from build123d import *

# Parameters (mm, degrees)
BOSS_EXTRUDE1_DEPTH = 1.6


with BuildPart() as part:
    # Эскиз1 → Повернуть1 (revolve)
    with BuildSketch(Plane.XY):
        Polygon((-2.875, 1.8), (0, 1.8), (0, -11.24), (-0.65, -11.9), (-1.195, -11.9), (-1.5, -11.595), (-1.5, -4.645), (-1.195, -4.34), (-1.195, 1), (-2.5, 1), (-2.5, 0), (-2.925, 0), (-2.925, 1.75), align=None)
    revolve(axis=Axis((0, 0, 0), (0, -1, 0)))

    # Sketch1 → Boss-Extrude1 (add)
    with BuildSketch(Plane(origin=(0, 1.8, 0), x_dir=(1, 0, 0), z_dir=(0, 1, 0))):
        Polygon((1.688749537, 2.925), (-1.688749537, 2.925), (-3.377499075, 0), (-1.688749537, -2.925), (1.688749537, -2.925), (3.377499075, 0), align=None)
    extrude(amount=-BOSS_EXTRUDE1_DEPTH)


solid = part.part
Verification items for the finished model (mm, model axes). A direction names the side the tool comes from. Coordinates: 2 decimals unless noted, no trailing zeros. Order: outer loops, then holes, each group sorted by start corner. A loop starts at its lowest first (then second) coordinate and runs counter-clockwise, first axis right, second up. Notation, with made-up numbers: (-26, -14.5) -> (21, -14.5) arc R19 ccw to (21, 4.5) -> close; hole circle Ø7 at (11, -26). An arc over 180 degrees is marked (long way). Put each result on its own line as item: value. Start each with the question number.
1. Material ranges on L1, parallel to X at y = 0.1, z = 0 (3 decimals); L2, parallel to Y at x = -2.25, z = -1.4, recorded low to high. Write a range as [from, to].
2. Go/stop test with flat-tipped pins: pin 1 Ø4 at (x, y) = (-1, -6) entering from +Z; pin 2 Ø1.6 at (x, z) = (1.5, 2.5) entering from -Y; pin 3 Ø1 at (x, y) = (1, -10) entering from +Z. Record where each tip stops, or that it passes through.
3. Mould release check, pull along X, two halves, no side actions. Record for faces 6 (the cylindrical face through (1.5, -8.07, -0.07)), 7 (the flat face through (2.545, 1.011, -1.442)), 8 (the flat face through (0, 1.8, 0)), 9 (the conical face through (0.15, -11.43, 0.11)): released by +X, released by -X, zero draft, split by the parting line, or undercut.
4. Cross-section at A-A, the plane x = -2. Record the boundary of the cut face in (y, z), then the cut area to 3 significant figures.
5. Access from +Z, -Z, +X, -X, +Y, -Y to the whole of each face (thin tool, end or side, straight path). Record for faces 1 (the flat face through (-1.5, 0.2, 2.7)), 2 (the flat face through (-2.545, 1.011, 1.442)), 3 (the flat face through (-1.5, 0.2, -2.7)), 4 (the flat face through (1.5, 0.2, 2.7)), 5 (the flat face through (1.5, 0.2, -2.7)).
6. Cross-section at D-D, the plane x = -2.75. Record the boundary of the cut face in (y, z).
7. Cross-section at B-B, the plane z = 2.2. Record the boundary of the cut face in (x, y).
8. Cross-section at C-C, the plane y = -4. Record the boundary of the cut face in (x, z) (3 decimals), then the cut area to 3 significant figures.
Computed:
1. L1: [-2.925, -2.5], [-1.195, 1.195], [2.5, 2.925]
1. L2: [0, 1.8]
2. pin 1: z = 1.5
2. pin 2: y = 0
2. pin 3: z = 1.41
3. face 6: split by the parting line
3. face 7: released by +X
3. face 8: zero draft
3. face 9: undercut
4. outline: (0, -2.13) -> (0.2, -2.13) -> (0.2, -2.39) -> (1.8, -2.39) -> (1.8, 2.39) -> (0.2, 2.39) -> (0.2, 2.13) -> (0, 2.13) -> (0, 1.5) -> (0.2, 1.5) -> (0.2, -1.5) -> (0, -1.5) -> close
4. area: 7.89 mm2
5. face 1: +Z, -X, -Y
5. face 2: +Z, -X, +Y, -Y
5. face 3: -Z, -X, -Y
5. face 4: +Z, +X, -Y
5. face 5: -Z, +X, -Y
6. outline: (0, -1) -> (0.2, -1) -> (0.2, -1.09) -> (1.8, -1.09) -> (1.8, 1.09) -> (0.2, 1.09) -> (0.2, 1) -> (0, 1) -> close
7. outline: (-2.11, 0.2) -> (-1.93, 0.2) -> (-1.93, 0) -> (-1.19, 0) -> (-1.19, 0.2) -> (1.19, 0.2) -> (1.19, 0) -> (1.93, 0) -> (1.93, 0.2) -> (2.11, 0.2) -> (2.11, 1.8) -> (-2.11, 1.8) -> close
8. outline: circle Ø2.39 at (0, 0)
8. area: 4.49 mm2
